Read the model definition and answer for the solid it produces. Units are mm, in the model's axes. A direction names the side the tool comes from. Round coordinates to 2 decimals unless told otherwise and drop trailing zeros. Write each loop counter-clockwise with the first axis right and the second up, starting at its lowest first coordinate (ties: lowest second). Pieces come first, ordered by that corner, then holes. Notation, with made-up numbers: (30, 85.5) -> (38, 85.5) arc R17 cw to (38, 96.5) -> close; hole circle Ø10 at (25.25, 5). An arc over 180 degrees is marked (long way). Return JSON: item names as keys, results as strings. Group by question number.
(1) Given pin 1 (12 mm diameter, centred on x = 7.5, z = -55.5, fed in from -Y), flat-ended and moving along its own axis, determine where the tip first touches the part or whether it passes through.
(2) For faces 1 (the flat face through (30.001, 43, -35)), 2 (the cylindrical face through (0.493, 32.066, -35.89)), determine the directions among +Z, -Z, +X, -X, +Y, -Y from which every point of the face is accessible in a straight line to the end or side of a thin tool.
(3) Straight lines are drawn through the part: line 1 (X direction, y = 52, z = -39.5); line 2 (Y direction, x = 12.5, z = -31.5). For each, find the intervals that lie inside material, in ascending order.
(4) A cutting plane is placed at C-C on z = -66. Give the vertices of the cut face in (x, y), then the cut area to 3 significant figures.
(5) The mould has two halves that part along Z. Classify faces 3 (the flat face through (15, 54.276, -53)), 4 (the cylindrical face through (21.194, 54.769, -82.805)), 5 (the cylindrical face through (30.493, 30.778, -35.697)): released by +Z, released by -Z, zero draft, split by the parting line, or undercut.
(6) A cutting plane is placed at B-B on y = 52.25. Give the vertices of the cut face in (x, z), then the cut area to 3 significant figures.
(7) A cutting plane is placed at D-D on x = 21.5. Give the vertices of the cut face in (y, z), then the cut area to 3 significant figures.
(8) A cutting plane is placed at A-A on x = 15.5. Give the vertices of the cut face in (y, z), then the cut area to 3 significant figures.
```python
from build123d import *

# Parameters (mm, degrees)
SKETCH1_R           = 0.8
SKETCH1_R_2         = 3
BOSS_EXTRUDE1_DEPTH = 31
BOSS_EXTRUDE2_DEPTH = 1
SKETCH5_R           = 0.8
CUT_EXTRUDE3_DEPTH  = 1
SKETCH5_3_R         = 3
CUT_EXTRUDE4_DEPTH  = 1
CUT_EXTRUDE5_START  = -1
CUT_EXTRUDE5_DEPTH  = 100.186902849


with BuildPart() as part:
    # Sketch1 → Boss-Extrude1 (new body)
    with BuildSketch(Plane(origin=(0, 0, 0), x_dir=(0, 0, -1), z_dir=(1, 0, 0))):
        with BuildLine():
            Line((27.520646447, 38.775594), (27.520646447, 55.275594))
            Line((27.520646447, 55.275594), (43.520646447, 55.275594))
            Line((43.520646447, 55.275594), (43.520646447, 38.775594))
            ThreePointArc((43.520646447, 38.775594), (35.520646447, 30.775594), (27.520646447, 38.775594))
        make_face()
        with Locations((35.520646447, 44.775594)):
            Circle(SKETCH1_R, mode=Mode.SUBTRACT)
        with Locations((41.515881392, 38.775594)):
            Circle(SKETCH1_R, mode=Mode.SUBTRACT)
        with Locations((35.520646447, 32.775594)):
            Circle(SKETCH1_R, mode=Mode.SUBTRACT)
        with Locations((29.515881392, 38.775594)):
            Circle(SKETCH1_R, mode=Mode.SUBTRACT)
        with Locations((35.520646447, 38.775594)):
            Circle(SKETCH1_R_2, mode=Mode.SUBTRACT)
    extrude(amount=BOSS_EXTRUDE1_DEPTH)

    # Sketch4 → Boss-Extrude2 (add)
    with BuildSketch(Plane(origin=(0, 55.275594, 0), x_dir=(1, 0, 0), z_dir=(0, 1, 0))):
        with BuildLine():
            Line((0, 43.520646447), (31, 43.520646447))
            Line((31, 43.520646447), (28.991162523, 45.242931174))
            ThreePointArc((28.991162523, 45.242931174), (26.414616828, 48.656689929), (25.5, 52.83470532))
            Line((25.5, 52.83470532), (25.5, 82.06609312))
            ThreePointArc((25.5, 82.06609312), (15.5, 92.06609312), (5.5, 82.06609312))
            Line((5.5, 82.06609312), (5.5, 52.83470532))
            ThreePointArc((5.5, 52.83470532), (4.585383172, 48.656689929), (2.008837477, 45.242931174))
            Line((2.008837477, 45.242931174), (0, 43.520646447))
        make_face()
    extrude(amount=-BOSS_EXTRUDE2_DEPTH)

    # Sketch5 → Cut-Extrude3 (cut)
    with BuildSketch(Plane.XZ.offset(-54.275594)):
        with Locations(Location((9.5, -82.06609312, 0), (0, 0, 270))):
            Circle(SKETCH5_R)
        with Locations(Location((15.5, -75.236093118, 0), (0, 0, 270))):
            Circle(SKETCH5_R)
        with Locations(Location((21.5, -82.06609312, 0), (0, 0, 270))):
            Circle(SKETCH5_R)
        with Locations(Location((15.5, -87.236093118, 0), (0, 0, 270))):
            Circle(SKETCH5_R)
    extrude(amount=-CUT_EXTRUDE3_DEPTH, mode=Mode.SUBTRACT)

    # Sketch5_3 → Cut-Extrude4 (cut)
    with BuildSketch(Plane.XZ.offset(-54.275594)):
        with Locations(Location((15.5, -82.06609312, 0), (0, 0, 270))):
            Circle(SKETCH5_3_R)
    extrude(amount=-CUT_EXTRUDE4_DEPTH, mode=Mode.SUBTRACT)

    # Sketch6 → Cut-Extrude5 (cut, through all)
    with BuildSketch(Plane(origin=(0, 55.275594, 0), x_dir=(1, 0, 0), z_dir=(0, 1, 0)).offset(CUT_EXTRUDE5_START)):
        Polygon((0.999214172, 43.494699328), (0.999214172, 44.172026991), (30.000785828, 44.172026991), (30.000785828, 43.494699328), (30.000785828, 27.546593566), (30.000785828, 27.028954782), (0.999214172, 27.028954782), (0.999214172, 27.546593566), align=None)
    extrude(amount=-CUT_EXTRUDE5_DEPTH, mode=Mode.SUBTRACT)


solid = part.part
```
Checks:
{
 "1": {"pin 1": "stops at y = 54.28"},
 "2": {"face 1": "+Z, -Z, -Y", "face 2": "+X, -X"},
 "3": {"line 1": "x = 0 to 1, 30 to 31", "line 2": "y = 54.28 to 55.28"},
 "4": {"outline": "(5.5, 54.28) -> (25.5, 54.28) -> (25.5, 55.28) -> (5.5, 55.28) -> close", "area": "20.0 mm^2"},
 "5": {"face 3": "zero draft", "face 4": "undercut", "face 5": "split by the parting line"},
 "6": {"outline": "(0, -43.52) -> (1, -43.52) -> (1, -27.52) -> (0, -27.52) -> close; (30, -43.52) -> (31, -43.52) -> (31, -27.52) -> (30, -27.52) -> close", "area": "32.0 mm^2"},
 "7": {"outline": "(54.28, -90.07) -> (55.28, -90.07) -> (55.28, -82.87) -> (54.28, -82.87) -> close; (54.28, -81.27) -> (55.28, -81.27) -> (55.28, -27.52) -> (54.28, -27.52) -> close", "area": "60.9 mm^2"},
 "8": {"outline": "(54.28, -92.07) -> (55.28, -92.07) -> (55.28, -88.04) -> (54.28, -88.04) -> close; (54.28, -86.44) -> (55.28, -86.44) -> (55.28, -85.07) -> (54.28, -85.07) -> close; (54.28, -79.07) -> (55.28, -79.07) -> (55.28, -76.04) -> (54.28, -76.04) -> close; (54.28, -74.44) -> (55.28, -74.44) -> (55.28, -27.52) -> (54.28, -27.52) -> close", "area": "55.3 mm^2"}
}
